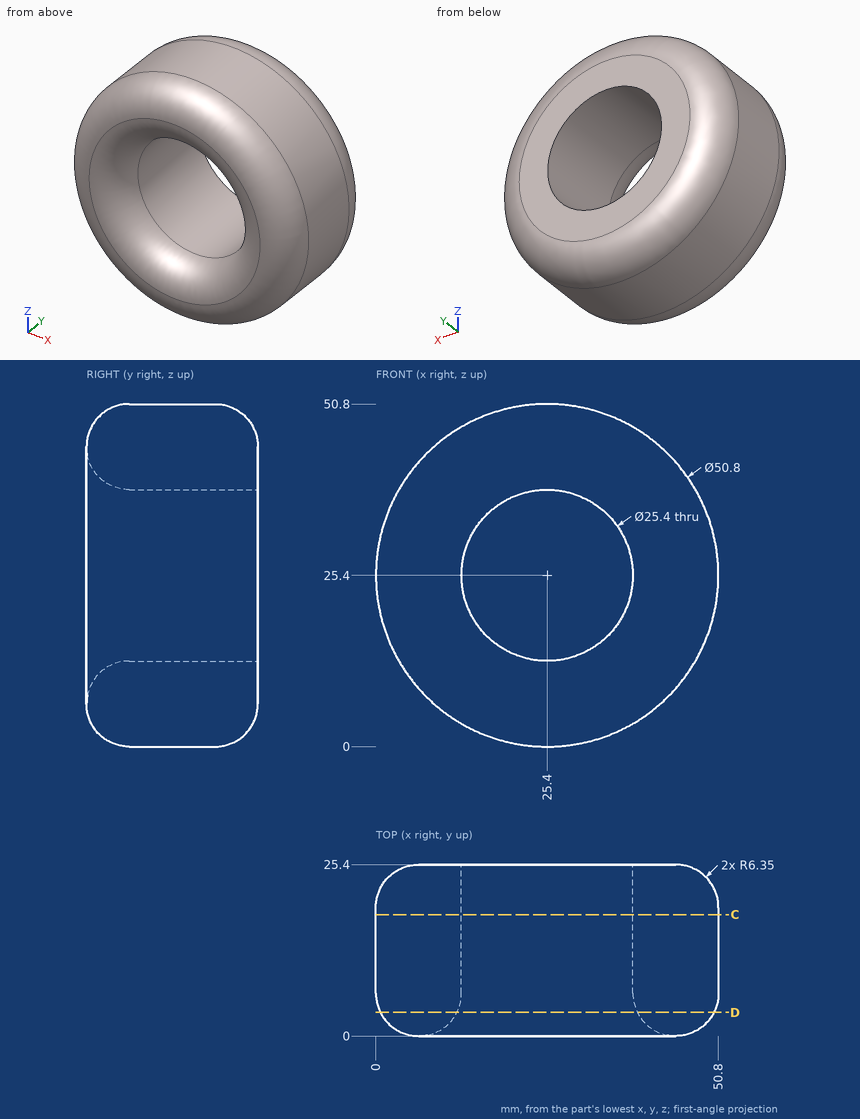
Print and shaded views of the part. All mm, measured from the part's lowest x, y and z. Give positions to 0.01 mm unless a question says otherwise; leave off trailing zeros. Loops run counter-clockwise (first coordinate to the right, second up) from the corner with the lowest first, then second, coordinate; pieces in that order, holes last.
1) Wall check: line 1 (Z direction, x = 25.4, y = 14); line 2 (X direction, y = 16.5, z = 25); line 3 (Z direction, x = 36, y = 14) (1 decimal). Give the ranges that are in metal, low to high.
2) Flat gauge pins, fed straight in: pin 1 Ø4 at (y, z) = (10, 9) entering from +X; pin 2 Ø20.5 at (x, z) = (25.4, 25.4) entering from +Y; pin 3 Ø5 at (x, y) = (6.5, 13) entering from +Z; pin 4 Ø4 at (y, z) = (4.5, 45.5) entering from +X. Where does each tip first touch, or does it go through?
3) Saw through at C-C (y = 18). Write the cut outline in (x, z).
4) Saw through at D-D (y = 3.5). Write the cut outline in (x, z), plus the area to 3 significant figures.
Answer block:
1. line 1: z = 0 to 12.7, 38.1 to 50.8
1. line 2: x = 0 to 12.71, 38.09 to 50.8
1. line 3: z = 2.3 to 18.4, 32.4 to 48.5
2. pin 1: stops at x = 46.32
2. pin 2: passes through
2. pin 3: stops at z = 44.8
2. pin 4: stops at x = 42.95
3. outline: circle Ø50.8 at (25.4, 25.4); hole circle Ø25.4 at (25.4, 25.4)
4. outline: circle Ø49.45 at (25.4, 25.4); hole circle Ø26.75 at (25.4, 25.4)
4. area: 1,360 mm2
